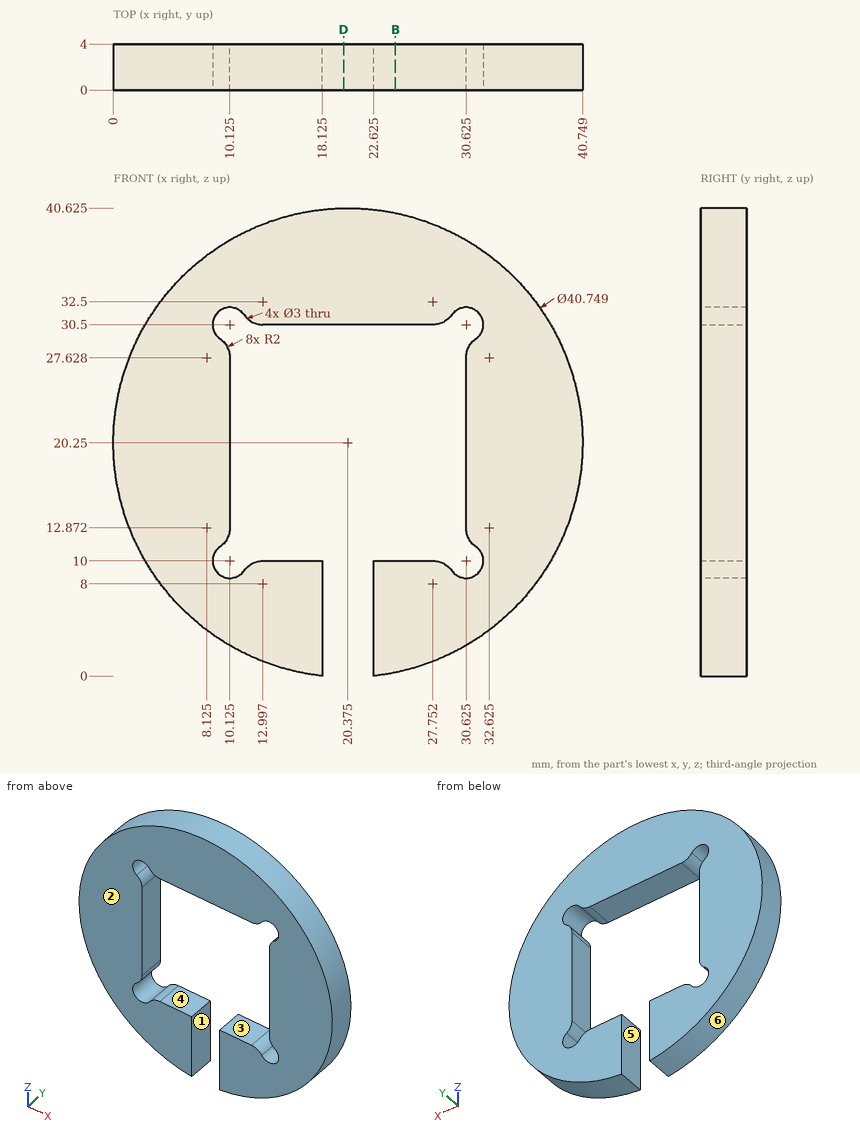
Could you check a few things on this drawing? It's one solid part, dimensions in mm from its lowest x, y, z. A direction names the side the tool comes from. Round coordinates to 2 decimals unless told otherwise and drop trailing zeros. Loops run counter-clockwise (first coordinate to the right, second up) from the corner with the lowest first, then second, coordinate; pieces in that order, holes last.
Q1. I want a section at D-D (x = 20). Write out the boundary of the cut face in (y, z).
Q2. Thinking about a two-plate mould opening in Z: for the marked faces 4, 5 and 6, which applies, pulls with the +Z half, pulls with the -Z half, needs draft (parallel to the pull), parting line crosses it, or undercut?
Q3. For P1, Ø2, axis at x = 8.5, y = 3.5, coming from the -Z side; P2, Ø1.5, axis at y = 1.5, z = 10.5, coming from the -X side (1 decimal); P3, Ø1, axis at x = 24, y = 1.5, coming from the +Z side; P4, Ø2.5, axis at x = 10.12, z = 10, coming from the +Y side, each with a flat end and sliding along its axis, tell me the tip position at first contact or that it passes through.
Q4. Please list where these lines run through material, in increasing order: L1, parallel to X at y = 0.4, z = 19 (1 decimal); L2, parallel to Z at x = 32, y = 1.85 (1 decimal); L3, parallel to X at y = 1.7, z = 14.5 (1 decimal).
Q5. I want a section at B-B (x = 24.5). Write out the boundary of the cut face in (y, z).
Q6. On a 3-axis mill with a long thin cutter (end or side, diameter ignored), from which of +Z, -Z, +X, -X, +Y, -Y can I reach the whole of each face in a straight line? I mean the marked faces 1, 2 and 3. Say none if no direction works.
Answer below:
1. outline: (0, 30.5) - (4, 30.5) - (4, 40.62) - (0, 40.62) - close
2. face 4: undercut
2. face 5: needs draft
2. face 6: parting line crosses it
3. P1: stops at z = 3.02
3. P2: stops at x = 2.1
3. P3: stops at z = 40.38
3. P4: passes through
4. L1: x = 0 to 10.1, 30.6 to 40.7
4. L2: z = 3.5 to 9.4, 10.6 to 29.9, 31.1 to 37
4. L3: x = 0.8 to 10.1, 30.6 to 39.9
5. outline: (0, 0.3) - (4, 0.3) - (4, 10) - (0, 10) - close; (0, 30.5) - (4, 30.5) - (4, 40.2) - (0, 40.2) - close
6. face 1: -Z, +Y, -Y
6. face 2: +Z, -Z, +X, -X, -Y
6. face 3: +Y, -Y
